from build123d import *

# Parameters (mm, degrees)
SKETCH1_R           = 1.5
SKETCH1_W           = 19.6
SKETCH1_H           = 45.1
BOSS_EXTRUDE1_DEPTH = 5
CUT_EXTRUDE2_DEPTH  = 5
SKETCH2_W           = 35
SKETCH2_H           = 97
CUT_EXTRUDE1_DEPTH  = 3


with BuildPart() as part:
    # Sketch1 → Boss-Extrude1 (new body)
    with BuildSketch(Plane(origin=(0, 0, 0), x_dir=(1, 0, 0), z_dir=(0, 1, 0))):
        Polygon((-59.213749531, -30), (-70, -13.390630812), (-70, 23.338095117), (-23.338095117, 70), (0, 70), (0, -30), align=None)
        with Locations((-43.840620434, 43.840620434)):
            Circle(SKETCH1_R, mode=Mode.SUBTRACT)
        with Locations((-63.979633983, -15.316867676)):
            Circle(SKETCH1_R, mode=Mode.SUBTRACT)
        with Locations((-37.8, 7.55)):
            Rectangle(SKETCH1_W, SKETCH1_H, mode=Mode.SUBTRACT)
    boss_extrude1 = extrude(amount=BOSS_EXTRUDE1_DEPTH)

    # Sketch3 → Cut-Extrude2 (cut)
    with BuildSketch(Plane(origin=(0, 5, 0), x_dir=(1, 0, 0), z_dir=(0, 1, 0))):
        Polygon((-20, -30), (-30, -20), (-65.707825463, -20), (-70, -13.390630812), (-52.6, 4.009369188), (-52.6, 40.738095117), (-43.338095117, 50), (-33.338095117, 50), (-28.338095117, 55), (-28.338095117, 65), (-75, 65), (-75, -30), align=None)
    cut_extrude2 = extrude(amount=-CUT_EXTRUDE2_DEPTH, mode=Mode.SUBTRACT)

    # Mirror1: Boss-Extrude1, Cut-Extrude2 across plane
    add(boss_extrude1.mirror(Plane(origin=(0, 5, 30), x_dir=(0, 0, 1), z_dir=(-1, 0, 0))))
    add(cut_extrude2.mirror(Plane(origin=(0, 5, 30), x_dir=(0, 0, 1), z_dir=(-1, 0, 0))), mode=Mode.SUBTRACT)

    # Sketch2 → Cut-Extrude1 (cut)
    with BuildSketch(Plane(origin=(0, 5, 0), x_dir=(1, 0, 0), z_dir=(0, 1, 0))):
        with Locations((0, 21.5)):
            Rectangle(SKETCH2_W, SKETCH2_H)
    extrude(amount=-CUT_EXTRUDE1_DEPTH, mode=Mode.SUBTRACT)


solid = part.part
Could you check a few things on this model? Use its own coordinates, in mm. A direction names the side the tool comes from. Coordinates: 2 decimals unless noted, no trailing zeros. Order: outer loops, then holes, each group sorted by start corner. A loop starts at its lowest first (then second) coordinate and runs counter-clockwise, first axis right, second up. Notation, with made-up numbers: (-6, 51) - (47, 51) arc R22 cw to (47, 67) - close; hole circle Ø3 at (61.5, 44.25). An arc over 180 degrees is marked (long way). Answer in a Markdown table with one row per item. Add a question column.
(1) I need wall thicknesses on L1, parallel to X at y = 1.55, z = -16.5; L2, parallel to X at y = 3.95, z = -5; L3, parallel to X at y = 3.25, z = -62. Which ranges of each line are inside material? Lowest first, please.
(2) On a 3-axis mill with a long thin cutter (end or side, diameter ignored), from which of +Z, -Z, +X, -X, +Y, -Y can I reach the whole of each face in a straight line? I mean faces 4 (the face through (38, 2, 15)), 5 (the face through (28.338, 3, -60)), 6 (the face through (-38, 3, -50)), 7 (the face through (-67.824, 2.465, 16.742)), 8 (the face through (17.5, 4, -21)). Say none if no direction works.
(3) Will these pins go through, and if not, where does the flat tip stop? pin 1 (1.5 mm diameter, centred on y = 3, z = -14.5, fed in from -X); pin 2 (1 mm diameter, centred on x = 28.5, y = 2, fed in from +Z); pin 3 (2.5 mm diameter, centred on x = -38, y = 3, fed in from -Z).
(4) If we section it at B-B, the plane z = -59: Please give me the cut outline in (x, y).
(5) If we section it at D-D, the plane y = 1.05: State how many separate pieces and enclosed holes the cut face has, then the cut area to 3 significant figures.
(6) If we section it at C-C, the plane x = 31.5: Please give me the cut outline in (y, z), then the cut area to 3 significant figures.
(7) If we mould it in two halves opening along Z, with no side actions, what happens to faces 1 (the face through (67.824, 2.465, 16.742)), 2 (the face through (42.41, 2.46, -44.29)), 3 (the face through (-61.42, 2.54, 4.81))? For each: released by +Z, released by -Z, zero draft, split by the parting line, or undercut.
(8) If we section it at A-A, the plane z = -18: Please give me the cut outline in (x, y).
Results are:
| question | item | result |
|---|---|---|
| 1 | L1 | x = -52.6 to -47.6, -28 to 28, 47.6 to 52.6 |
| 1 | L2 | x = -52.6 to -47.6, -28 to -17.5, 17.5 to 28, 47.6 to 52.6 |
| 1 | L3 | x = -28.34 to -17.5, 17.5 to 28.34 |
| 2 | face 4 | +Y, -Y |
| 2 | face 5 | -Z, +X, +Y, -Y |
| 2 | face 6 | -Z, -X, +Y, -Y |
| 2 | face 7 | +Z, -X, +Y, -Y |
| 2 | face 8 | -Z, +Y |
| 3 | pin 1 | stops at x = -52.6 |
| 3 | pin 2 | stops at z = 22 |
| 3 | pin 3 | stops at z = -50 |
| 4 | outline | (-28.34, 0) - (28.34, 0) - (28.34, 5) - (17.5, 5) - (17.5, 2) - (-17.5, 2) - (-17.5, 5) - (-28.34, 5) - close |
| 5 | separate pieces | 1 |
| 5 | enclosed holes | 6 |
| 5 | area | 7,620 mm2 |
| 6 | outline | (0, -51.84) - (5, -51.84) - (5, -30.1) - (0, -30.1) - close; (0, 15) - (5, 15) - (5, 20) - (0, 20) - close |
| 6 | area | 134 mm2 |
| 7 | face 1 | released by +Z |
| 7 | face 2 | undercut |
| 7 | face 3 | released by -Z |
| 8 | outline | (-52.6, 0) - (-47.6, 0) - (-47.6, 5) - (-52.6, 5) - close; (-28, 0) - (28, 0) - (28, 5) - (17.5, 5) - (17.5, 2) - (-17.5, 2) - (-17.5, 5) - (-28, 5) - close; (47.6, 0) - (52.6, 0) - (52.6, 5) - (47.6, 5) - close |
